Verification items for the finished model (mm, model axes). A direction names the side the tool comes from. Round coordinates to 2 decimals unless told otherwise and drop trailing zeros. Write each loop counter-clockwise with the first axis right and the second up, starting at its lowest first coordinate (ties: lowest second). Pieces come first, ordered by that corner, then holes. Notation, with made-up numbers: (58, -24.5) - (76, -24.5) arc R16 cw to (76, 1.5) - close; hole circle Ø7 at (26, 50.5). An arc over 180 degrees is marked (long way). Answer as a JSON object with one key per item and string values.
```python
from build123d import *

# Parameters (mm, degrees)
F0_W     = 508
F0_H     = 168.275
F1_DEPTH = 19.05
F2_W     = 19.05
F2_H     = 40.64
F2_H_2   = 34.925
F3_DEPTH = 25.4
F4_W     = 469.9
F4_H     = 19.05
F5_DEPTH = 15.875


with BuildPart() as f1:
    # F0 (on Right) → F1 (new body)
    with BuildSketch(Plane.YZ):
        with Locations((-3.356125, -38.352349)):
            Rectangle(F0_W, F0_H)
    extrude(amount=F1_DEPTH)

    # F2 (on face) → F3 (cut)
    with BuildSketch(Plane.YZ.offset(19.05)):
        with Locations((241.118875, 25.465151)):
            Rectangle(F2_W, F2_H)
        with Locations((241.118875, -55.814849)):
            Rectangle(F2_W, F2_H)
        with Locations((241.118875, -139.952349)):
            Rectangle(F2_W, F2_H_2)
        with Locations((-247.831125, -55.814849)):
            Rectangle(F2_W, F2_H)
        with Locations((-247.831125, 25.465151)):
            Rectangle(F2_W, F2_H)
    extrude(amount=-F3_DEPTH, mode=Mode.SUBTRACT)

    # F4 (on face) → F5 (cut)
    with BuildSketch(Plane(origin=(0, 0, 0), x_dir=(0, -1, 0), z_dir=(-1, 0, 0))):
        with Locations((3.356125, 36.260151)):
            Rectangle(F4_W, F4_H)
    extrude(amount=-F5_DEPTH, mode=Mode.SUBTRACT)


solid = f1.part
```
1. Access from +Z, -Z, +X, -X, +Y, -Y to the whole of each face (thin tool, end or side, straight path). Record for faces 1 (the face through (10, 241, -35.495)), 2 (the face through (10, -248, -35.495)), 3 (the face through (8, 0, 26.735)), 4 (the face through (12, 231.594, 21)).
Completed:
{"face 1": "+X, -X, +Y", "face 2": "+X, -X, -Y", "face 3": "+Z, -X, +Y, -Y", "face 4": "+Z, +X, -X, +Y"}
2. Material ranges on probe 1 along Z at (x, y) = (1.5, -117); probe 2 along Y at (x, z) = (12, -50.5), recorded low to high. Write a range as from..to.
Completed:
{"probe 1": "z = -122.49..26.74", "probe 2": "y = -238.31..231.59"}
3. Go/stop test with flat-tipped pins: pin 1 (4 mm diameter, centred on y = -99, z = -99.5, fed in from -X); pin 2 (2 mm diameter, centred on x = 4, y = -146.5, fed in from +Z); pin 3 (9.5 mm diameter, centred on x = 11.5, z = -58, fed in from -Y); pin 4 (9.5 mm diameter, centred on y = -1, z = 33, fed in from -X) (3 decimals). Record where each tip stops, or that it passes through.
Completed:
{"pin 1": "stops at x = 0", "pin 2": "stops at z = 26.74", "pin 3": "stops at y = -238.31", "pin 4": "stops at x = 15.875"}
4. Cross-section at A-A (x = 11.5). Record the boundary of the cut face in (y, z).
Completed:
{"outline": "(-257.36, -122.49) - (250.64, -122.49) - (250.64, -76.13) - (231.59, -76.13) - (231.59, -35.49) - (250.64, -35.49) - (250.64, 5.15) - (231.59, 5.15) - (231.59, 26.74) - (-238.31, 26.74) - (-238.31, 5.15) - (-257.36, 5.15) - (-257.36, -35.49) - (-238.31, -35.49) - (-238.31, -76.13) - (-257.36, -76.13) - close"}
5. Cross-section at C-C (z = 14). Record the boundary of the cut face in (x, y), plus the area to 3 significant figures.
Completed:
{"outline": "(0, -238.31) - (19.05, -238.31) - (19.05, 231.59) - (0, 231.59) - close", "area": "8,950 mm^2"}
6. Cross-section at B-B (y = 90.5). Record the boundary of the cut face in (x, z) (3 decimals), plus the area to 3 significant figures.
Completed:
{"outline": "(0, -122.49) - (19.05, -122.49) - (19.05, 45.785) - (15.875, 45.785) - (15.875, 26.735) - (0, 26.735) - close", "area": "2,900 mm^2"}
